The listing builds one solid part. Answer for the finished solid, in the listing's coordinates (mm). Coordinates: 2 decimals unless noted, no trailing zeros. Loops run counter-clockwise (first coordinate to the right, second up) from the corner with the lowest first, then second, coordinate; pieces in that order, holes last. Notation, with made-up numbers: (11.5, 31) - (60.5, 31) arc R18 ccw to (60.5, 49) - close; hole circle Ø3 at (75, -39). An arc over 180 degrees is marked (long way). Put each result on its own line as item: value.
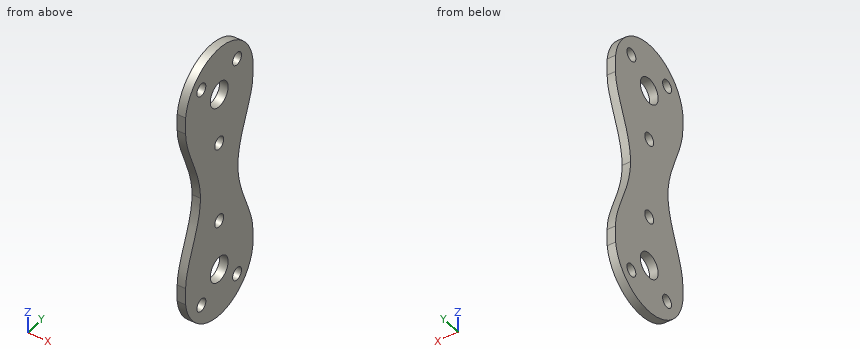
```python
from build123d import *

# Parameters (mm, degrees)
SCHIZZO1_R                   = 1.5
SCHIZZO1_R_2                 = 3
ESTRUSIONE_ESTRUSIONE1_DEPTH = 2


with BuildPart() as part:
    # Schizzo1 → Estrusione-Estrusione1 (new body)
    with BuildSketch(Plane(origin=(0, 0, 0), x_dir=(0, 0, -1), z_dir=(1, 0, 0))):
        with BuildLine():
            Line((-2.501010101, -11.3), (1.498989899, -11.3))
            ThreePointArc((1.498989899, -11.3), (11.398989899, 0), (1.498989899, 11.3))
            Line((1.498989899, 11.3), (-2.501010101, 11.3))
            add(Edge.make_bspline(
                [(-2.501010101, 11.3), (-7.839898951, 11.429610053), (-14.35178918, 6.216652626), (-21.601010101, 6.3)],
                knots=[0, 0, 0, 0, 1, 1, 1, 1], degree=3))
            add(Edge.make_bspline(
                [(-40.701010101, 11.3), (-35.362121251, 11.429610053), (-28.850231022, 6.216652626), (-21.601010101, 6.3)],
                knots=[0, 0, 0, 0, 1, 1, 1, 1], degree=3))
            Line((-40.701010101, 11.3), (-44.701010101, 11.3))
            ThreePointArc((-44.701010101, 11.3), (-54.601010101, 0), (-44.701010101, -11.3))
            Line((-44.701010101, -11.3), (-40.701010101, -11.3))
            add(Edge.make_bspline(
                [(-40.701010101, -11.3), (-34.455779635, -11.063584615), (-28.769360616, -6.33994929), (-21.601010101, -6.3)],
                knots=[0, 0, 0, 0, 1, 1, 1, 1], degree=3))
            add(Edge.make_bspline(
                [(-2.501010101, -11.3), (-8.746240567, -11.063584615), (-14.432659586, -6.33994929), (-21.601010101, -6.3)],
                knots=[0, 0, 0, 0, 1, 1, 1, 1], degree=3))
        make_face()
        with Locations((-48.202020202, 6)):
            Circle(SCHIZZO1_R, mode=Mode.SUBTRACT)
        with Locations((-48.202020202, -6)):
            Circle(SCHIZZO1_R, mode=Mode.SUBTRACT)
        with Locations((-31.202020202, 0)):
            Circle(SCHIZZO1_R, mode=Mode.SUBTRACT)
        with Locations((-12, 0)):
            Circle(SCHIZZO1_R, mode=Mode.SUBTRACT)
        with Locations((5, 6)):
            Circle(SCHIZZO1_R, mode=Mode.SUBTRACT)
        with Locations((5, -6)):
            Circle(SCHIZZO1_R, mode=Mode.SUBTRACT)
        with Locations((-43.202020202, 0)):
            Circle(SCHIZZO1_R_2, mode=Mode.SUBTRACT)
        Circle(SCHIZZO1_R_2, mode=Mode.SUBTRACT)
    extrude(amount=ESTRUSIONE_ESTRUSIONE1_DEPTH)


solid = part.part
```
1) Straight lines are drawn through the part: L1, parallel to Z at x = 1.7, y = 2; L2, parallel to Z at x = 0.85, y = -1.75; L3, parallel to Y at x = 1.05, z = -5. For each, find the intervals that lie inside material, in ascending order. Write a range as [from, to].
Found:
L1: z = [-11.22, -2.24], [2.24, 40.97], [45.44, 54.42]
L2: z = [-11.26, -2.44], [2.44, 40.77], [45.64, 54.47]
L3: y = [-10.24, -7.5], [-4.5, 4.5], [7.5, 10.24]
2) Each of these flat-tipped pins is pushed along its axis until it touches: pin 1 (4 mm diameter, centred on y = 6, z = -5, fed in from +X); pin 2 (5.5 mm diameter, centred on y = 0, z = 0, fed in from -X); pin 3 (1 mm diameter, centred on x = 1.5, z = 27, fed in from -Y); pin 4 (1 mm diameter, centred on x = 0.5, z = 43, fed in from +Y). Where does it stop, or does it pass through?
Found:
pin 1: stops at x = 2
pin 2: passes through
pin 3: stops at y = -7.29
pin 4: stops at y = 11.3
3) The part is cut by section B-B (z = 48.5). Give the vertices of the cut face in (x, y).
Found:
outline: (0, -10.09) - (2, -10.09) - (2, -7.47) - (0, -7.47) - close; (0, -4.53) - (2, -4.53) - (2, 4.53) - (0, 4.53) - close; (0, 7.47) - (2, 7.47) - (2, 10.09) - (0, 10.09) - close
4) The part is cut by section A-A (y = 0). Give the vertices of the cut face in (x, z), and give its area (3 significant figures).
Found:
outline: (0, -11.4) - (2, -11.4) - (2, -3) - (0, -3) - close; (0, 3) - (2, 3) - (2, 10.5) - (0, 10.5) - close; (0, 13.5) - (2, 13.5) - (2, 29.7) - (0, 29.7) - close; (0, 32.7) - (2, 32.7) - (2, 40.2) - (0, 40.2) - close; (0, 46.2) - (2, 46.2) - (2, 54.6) - (0, 54.6) - close
area: 96.0 mm^2
5) The part is cut by section C-C (z = 41.5). Give the vertices of the cut face in (x, y).
Found:
outline: (0, -11.3) - (2, -11.3) - (2, -2.47) - (0, -2.47) - close; (0, 2.47) - (2, 2.47) - (2, 11.3) - (0, 11.3) - close
6) The part is cut by section D-D (x = 0.8). State how many separate pieces and enclosed holes the cut face has, and give its area (3 significant figures).
Found:
separate pieces: 1
enclosed holes: 8
area: 1,080 mm^2
